```python
from build123d import *

# Parameters (mm, degrees)
F0_R        = 2
F0_W        = 6.25
F0_H        = 5.75
F1_DEPTH    = 13
F3_DEPTH    = 25
F4_T1_DEPTH = 35.5
F6_DEPTH    = 2.5
F7_T1_DEPTH = 15.9435440675


# Not quite as in the source:
# - a fillet or chamfer that OpenCascade refuses, or shapes differently, is made with other operations: its cross-section is extruded or revolved along the edge and cut away or added


with BuildPart() as f1:
    # F0 (on Front) → F1 (new body)
    with BuildSketch(Plane.XZ):
        Polygon((-8.25, 3.5), (-8.25, 5.25), (-14, 5.25), (-14, -5.25), (-8.25, -5.25), (-8.25, -2.25), (-6.25, -2.25), (-6.25, 3.5), align=None)
        with Locations((-10, 0)):
            Circle(F0_R, mode=Mode.SUBTRACT)
        with Locations((-10, 0)):
            Circle(F0_R)
        Polygon((0, 3.5), (0, 5.25), (-8.25, 5.25), (-8.25, 3.5), (-6.25, 3.5), align=None)
        with Locations((-3.125, 0.625)):
            Rectangle(F0_W, F0_H)
        Polygon((0, -5.25), (0, -2.25), (-6.25, -2.25), (-8.25, -2.25), (-8.25, -5.25), align=None)
    extrude(amount=F1_DEPTH)

    # F0 (on Front) → F2 (revolve, cut)
    with BuildSketch(Plane.XZ):
        Polygon((0, 3.5), (0, 5.25), (-8.25, 5.25), (-8.25, 3.5), (-6.25, 3.5), align=None)
        with Locations((-3.125, 0.625)):
            Rectangle(F0_W, F0_H)
        Polygon((0, -5.25), (0, -2.25), (-6.25, -2.25), (-8.25, -2.25), (-8.25, -5.25), align=None)
    revolve(axis=Axis((0, 0, 0), (0, 0, -1)), mode=Mode.SUBTRACT)

    # F0 (on Front) → F3 (cut)
    with BuildSketch(Plane.XZ):
        with Locations((-10, 0)):
            Circle(F0_R)
    extrude(amount=F3_DEPTH, mode=Mode.SUBTRACT)

    # F4: fillet of radius 5 on 1 edges, made by hand

    # F4_s2 → F4_t1 (cut)
    with BuildSketch(Plane.XY.offset(-17.75)):
        with BuildLine():
            ThreePointArc((-14, -8), (-12.5355339059, -11.5355339059), (-9, -13))
            Line((-9, -13), (-14, -13))
            Line((-14, -13), (-14, -8))
        make_face()
    extrude(amount=F4_T1_DEPTH, mode=Mode.SUBTRACT)

    # F5 (on face) → F6 (cut)
    with BuildSketch(Plane.XZ.offset(13)):
        with BuildLine():
            Line((-17.9225690663, -4), (-10, -4))
            ThreePointArc((-10, -4), (-12.8284271247, -2.8284271247), (-14, 0))
            Line((-14, 0), (-17.9225690663, 0))
            Line((-17.9225690663, 0), (-17.9225690663, -4))
        make_face()
        with BuildLine():
            ThreePointArc((-14, 0), (-12.8284271247, 2.8284271247), (-10, 4))
            Line((-10, 4), (-17.9225690663, 4))
            Line((-17.9225690663, 4), (-17.9225690663, 0))
            Line((-17.9225690663, 0), (-14, 0))
        make_face()
        with BuildLine():
            Line((-10, 0), (-10, 4))
            ThreePointArc((-10, 4), (-12.8284271247, 2.8284271247), (-14, 0))
            Line((-14, 0), (-10, 0))
        make_face()
        with BuildLine():
            ThreePointArc((-9, -3.8729833462), (-6.8377223398, -2.4494897428), (-6, 0))
            ThreePointArc((-6, 0), (-6.8377223398, 2.4494897428), (-9, 3.8729833462))
            Line((-9, 3.8729833462), (-9, 1.7320508076))
            ThreePointArc((-9, 1.7320508076), (-8.2679491924, 1), (-8, 0))
            ThreePointArc((-8, 0), (-8.2679491924, -1), (-9, -1.7320508076))
            Line((-9, -1.7320508076), (-9, -3.8729833462))
        make_face()
        with BuildLine():
            Line((-9, 1.7320508076), (-9, 3.8729833462))
            ThreePointArc((-9, 3.8729833462), (-9.4959828301, 3.9681187851), (-10, 4))
            Line((-10, 4), (-10, 0))
            Line((-10, 0), (-10, -4))
            ThreePointArc((-10, -4), (-9.4959828301, -3.9681187851), (-9, -3.8729833462))
            Line((-9, -3.8729833462), (-9, -1.7320508076))
            ThreePointArc((-9, -1.7320508076), (-8.2679491924, -1), (-8, 0))
            ThreePointArc((-8, 0), (-8.2679491924, 1), (-9, 1.7320508076))
        make_face()
        with BuildLine():
            ThreePointArc((-14, 0), (-12.8284271247, -2.8284271247), (-10, -4))
            Line((-10, -4), (-10, 0))
            Line((-10, 0), (-14, 0))
        make_face()
    extrude(amount=-F6_DEPTH, mode=Mode.SUBTRACT)

    # F7: chamfer of 1 on 2 edges, made by hand

    # F7_s2 → F7_t1 (cut)
    with BuildSketch(Plane.YZ.offset(-13.3718610795)):
        Polygon((-12, -5.25), (-13, -4.25), (-13, -5.25), align=None)
        Polygon((-12, 5.25), (-13, 4.25), (-13, 5.25), align=None)
    extrude(amount=F7_T1_DEPTH, mode=Mode.SUBTRACT)

    # F8: F1 across face


with BuildPart() as f1_1:
    add(f1.part)
    add(f1.part.mirror(Plane(origin=(0, -9.948326432, 0.119047619), x_dir=(0, 1, 0), z_dir=(1, 0, 0))))


solid = f1_1.part
```
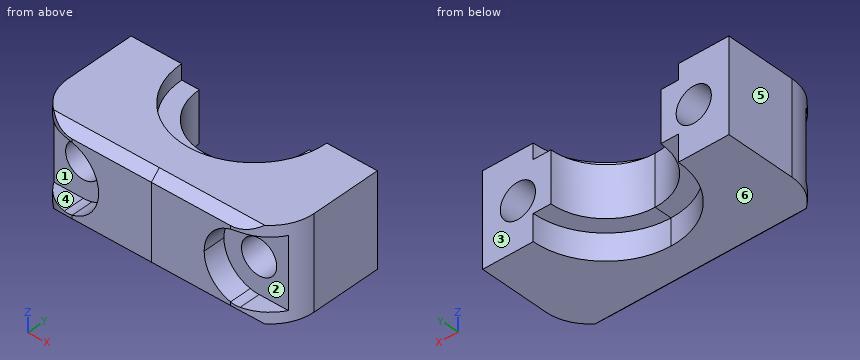
Here's how the part is built. I have some questions about the finished solid (model axes, mm). Face numbers are marked on the shaded views. A direction names the side the tool comes from. Give positions to 0.01 mm unless a question says otherwise; leave off trailing zeros. Write each loop counter-clockwise with the first axis right and the second up, starting at its lowest first coordinate (ties: lowest second). Pieces come first, ordered by that corner, then holes.
(1) Imagine slicing it at B-B, the plane x = -11. Write out the boundary of the cut face in (y, z).
Output values:
outline: (-12.58, -4.67) - (-12, -5.25) - (0, -5.25) - (0, -1.73) - (-10.5, -1.73) - (-10.5, -4) - (-12.58, -4) - close; (-12.58, 4) - (-10.5, 4) - (-10.5, 1.73) - (0, 1.73) - (0, 5.25) - (-12, 5.25) - (-12.58, 4.67) - close
(2) Imagine slicing it at A-A, the plane y = -1.5. Write out the boundary of the cut face in (x, z).
Output values:
outline: (-14, -5.25) - (-8.11, -5.25) - (-8.11, -2.25) - (-6.07, -2.25) - (-6.07, 3.5) - (-8.11, 3.5) - (-8.11, 5.25) - (-14, 5.25) - close; (6.07, -2.25) - (8.11, -2.25) - (8.11, -5.25) - (14, -5.25) - (14, 5.25) - (8.11, 5.25) - (8.11, 3.5) - (6.07, 3.5) - close; hole circle Ø4 at (-10, 0); hole circle Ø4 at (10, 0)
(3) Thinking about a two-plate mould opening in Z: for the marked faces 4, 5 and 6, which applies, pulls with the +Z half, pulls with the -Z half, needs draft (parallel to the pull), parting line crosses it, or undercut?
Output values:
face 4: undercut
face 5: needs draft
face 6: pulls with the -Z half
(4) Imagine slicing it at D-D, the plane y = -8.75. Write out the boundary of the cut face in (x, z), and give its area (3 significant figures).
Output values:
outline: (-13.94, -5.25) - (13.94, -5.25) - (13.94, 5.25) - (-13.94, 5.25) - close; hole circle Ø4 at (-10, 0); hole circle Ø4 at (10, 0)
area: 268 mm2
(5) If I drill on L1, parallel to Z at x = 11.5, y = -11; L2, parallel to X at y = -8.5, z = 1; L3, parallel to Z at x = 10, y = -3, over which ranges is the centre line in solid material (lowest first)?
Output values:
L1: z = -5.25 to -4, 4 to 5.25
L2: x = -13.97 to -11.73, -8.27 to 8.27, 11.73 to 13.97
L3: z = -5.25 to -2, 2 to 5.25
(6) On a 3-axis mill with a long thin cutter (end or side, diameter ignored), from which of +Z, -Z, +X, -X, +Y, -Y can I reach the whole of each face in a straight line? I mean the marked faces 1, 2 and 3. Say none if no direction works.
Output values:
face 1: -X, -Y
face 2: +X, -Y
face 3: +Z, -Z, +X, -X, +Y
(7) Will these pins go through, and if not, where does the flat tip stop? pin 1 (4 mm diameter, centred on x = 3, y = -4, fed in from -Z); pin 2 (3.5 mm diameter, centred on x = 10, z = -2, fed in from -Y).
Output values:
pin 1: stops at z = -2.25
pin 2: stops at y = -10.5
(8) Imagine slicing it at C-C, the plane z = 4.75. Write out the boundary of the cut face in (x, y).
Output values:
outline: (-14, -8) arc R5 ccw to (-11.18, -12.5) - (11.18, -12.5) arc R5 ccw to (14, -8) - (14, 0) - (8.25, 0) arc R8.25 cw to (-8.25, 0) - (-14, 0) - close
